Can you work these out from the model? Positions are in its coordinate system, mm. A direction names the side the tool comes from. Round coordinates to 2 decimals unless told otherwise and drop trailing zeros. Write each loop counter-clockwise with the first axis right and the second up, starting at its lowest first coordinate (ties: lowest second). Pieces come first, ordered by that corner, then holes. Notation, with made-up numbers: (-17.75, 31.5) -> (-3.75, 31.5) arc R19 cw to (-3.75, 67.5) -> close; hole circle Ø4 at (85, -25.75). An arc over 180 degrees is marked (long way). Write item = value, one per line. Start each with the question number.
1) For faces 1 (the face through (20.9, -9, -15)), 2 (the face through (-12.78, -8.6, -2.25)), 3 (the face through (-18.7, -9.64, -0.69)), which set-ups out of +Z, -Z, +X, -X, +Y, -Y let a thin tool reach every point of the face, with its end or its side?
2) If I drill on line 1 (X direction, y = -10, z = -13.5); line 2 (X direction, y = -9.5, z = -1.25); line 3 (Z direction, x = 20, y = -13.75), over which ranges is the centre line in solid material (lowest first)?
3) Imagine slicing it at A-A, the plane x = -12.95. Please give me the cut outline in (y, z).
4) I'm going to push a flat-ended pin straight in: pin 1 (5 mm diameter, centred on x = -11.5, z = -17.5, fed in from +Y). Where does the tip first touch, or does it pass through?
5) Imagine slicing it at C-C, the plane z = -4.75. State how many separate pieces and enclosed holes the cut face has, then the cut area to 3 significant figures.
6) Thinking about a two-plate mould opening in X: for faces 4 (the face through (-24.404, -10, -10)), 5 (the face through (0, -14.4, -9)), 6 (the face through (-13, -12.4, -19)), which applies, +X half, -X half, draft (parallel to the pull), parting line (faces both ways), or undercut?
7) Imagine slicing it at B-B, the plane y = -9.25. Please give me the cut outline in (x, z), then the cut area to 3 significant figures.
from build123d import *

# Parameters (mm, degrees)
SALIENTE_EXTRUIR1_DEPTH = 7.5
CROQUIS3_W              = 48.808095268
CROQUIS3_H              = 21.684781413
SALIENTE_EXTRUIR2_DEPTH = 2
CROQUIS4_R              = 7.95
CORTAR_EXTRUIR1_DEPTH   = 3
CORTAR_EXTRUIR1_TAPER   = -30
CORTAR_EXTRUIR2_DEPTH   = 4


with BuildPart() as part:
    # Croquis2 → Saliente-Extruir1 (new body)
    with BuildSketch(Plane(origin=(0, -4.9, 0), x_dir=(-1, 0, 0), z_dir=(0, -1, 0))):
        with BuildLine():
            Line((-5, 20.4), (5, 20.4))
            Line((5, 20.4), (5, 10.2))
            ThreePointArc((5, 10.2), (12.95, 2.25), (20.9, 10.2))
            Line((20.9, 10.2), (20.9, 20.4))
            Line((20.9, 20.4), (24.404047634, 20.4))
            Line((24.404047634, 20.4), (24.404047634, -1.284781413))
            Line((24.404047634, -1.284781413), (-24.404047634, -1.284781413))
            Line((-24.404047634, -1.284781413), (-24.404047634, 20.4))
            Line((-24.404047634, 20.4), (-20.9, 20.4))
            Line((-20.9, 20.4), (-20.9, 10.2))
            ThreePointArc((-20.9, 10.2), (-12.95, 2.25), (-5, 10.2))
            Line((-5, 10.2), (-5, 20.4))
        make_face()
    extrude(amount=SALIENTE_EXTRUIR1_DEPTH)

    # Croquis3 → Saliente-Extruir2 (add)
    with BuildSketch(Plane.XZ.offset(12.4)):
        with Locations((0, -9.557609294)):
            Rectangle(CROQUIS3_W, CROQUIS3_H)
    extrude(amount=SALIENTE_EXTRUIR2_DEPTH)

    # Croquis4 → Cortar-Extruir1 (cut)
    with BuildSketch(Plane.XZ.offset(12.4)):
        with Locations((-12.95, -10.2)):
            Circle(CROQUIS4_R)
        with Locations((12.95, -10.2)):
            Circle(CROQUIS4_R)
    extrude(amount=CORTAR_EXTRUIR1_DEPTH, taper=CORTAR_EXTRUIR1_TAPER, mode=Mode.SUBTRACT)

    # Croquis7 → Cortar-Extruir2 (cut)
    with BuildSketch(Plane.XY.offset(1.284781413)):
        with BuildLine():
            Line((-21.373206473, -7.088443063), (-21.373206473, -13.188443063))
            Line((-21.373206473, -13.188443063), (-17.173206473, -13.188443063))
            Line((-17.173206473, -13.188443063), (-20.273206473, -5.988443063))
            ThreePointArc((-20.273206473, -5.988443063), (-21.051023932, -6.310625604), (-21.373206473, -7.088443063))
        make_face()
        with BuildLine():
            Line((21.373206473, -13.188443063), (17.173206473, -13.188443063))
            Line((17.173206473, -13.188443063), (20.273206473, -5.988443063))
            ThreePointArc((20.273206473, -5.988443063), (21.051023932, -6.310625604), (21.373206473, -7.088443063))
            Line((21.373206473, -7.088443063), (21.373206473, -13.188443063))
        make_face()
    extrude(amount=-CORTAR_EXTRUIR2_DEPTH, mode=Mode.SUBTRACT)


solid = part.part
Reported:
q1.face_1 = -Z, +Y
q1.face_2 = -Z, +Y, -Y
q1.face_3 = +Z
q2.line_1 = -24.4 to -20.9, -5 to 5, 20.9 to 24.4
q2.line_2 = -24.4 to -21.37, -18.76 to 18.76, 21.37 to 24.4
q2.line_3 = -20.4 to -15.35, -5.05 to 1.28
q3.outline = (-14.4, -20.4) -> (-12.4, -20.4) -> (-12.4, -18.15) -> (-14.4, -19.3) -> close; (-14.4, -1.1) -> (-12.4, -2.25) -> (-4.9, -2.25) -> (-4.9, 1.28) -> (-14.4, 1.28) -> close
q4.pin_1 = -12.4
q5.separate_pieces = 3
q5.enclosed_holes = 0
q5.area = 238 mm²
q6.face_4 = -X half
q6.face_5 = draft
q6.face_6 = undercut
q7.outline = (-24.4, -20.4) -> (-20.9, -20.4) -> (-20.9, -10.2) arc R7.95 cw to (-5, -10.2) -> (-5, -20.4) -> (5, -20.4) -> (5, -10.2) arc R7.95 cw to (20.9, -10.2) -> (20.9, -20.4) -> (24.4, -20.4) -> (24.4, 1.28) -> (21.37, 1.28) -> (21.37, -2.72) -> (18.87, -2.72) -> (18.87, 1.28) -> (-18.87, 1.28) -> (-18.87, -2.72) -> (-21.37, -2.72) -> (-21.37, 1.28) -> (-24.4, 1.28) -> close
q7.area = 515 mm²
